```python
from build123d import *

# Parameters (mm, degrees)
RESSALTO_EXTRUS_O1_DEPTH = 12.5


with BuildPart() as part:
    # Esboço1 → Ressalto-extrusão1 (new body)
    with BuildSketch(Plane.XY):
        with BuildLine():
            Line((10, -22.912878475), (10, -17.320508076))
            ThreePointArc((10, -17.320508076), (-19.318516526, -5.176380902), (0, 20))
            Line((0, 20), (0, 40))
            ThreePointArc((0, 40), (-2.5, 42.5), (-5, 40))
            Line((-5, 40), (-4.923076923, 39.384615385))
            Line((-4.923076923, 39.384615385), (-2.728764161, 21.830113288))
            ThreePointArc((-2.728764161, 21.830113288), (-21.36959311, 5.228813472), (-12.5, -18.10386699))
            Line((-12.5, -18.10386699), (-12.5, -21.650635095))
            ThreePointArc((-12.5, -21.650635095), (-1.400290894, -24.960752902), (10, -22.912878475))
        make_face()
    extrude(amount=RESSALTO_EXTRUS_O1_DEPTH)


solid = part.part
```
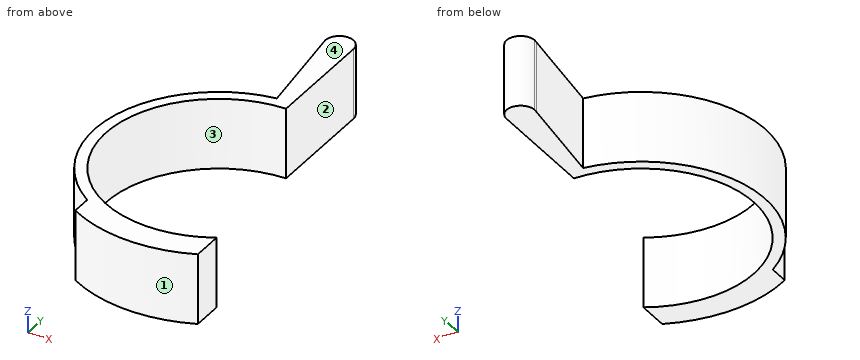
Read the model definition and answer for the solid it produces. Units are mm, in the model's axes. Face numbers are marked on the shaded views. Give positions to 0.01 mm unless a question says otherwise; leave off trailing zeros. Loops run counter-clockwise (first coordinate to the right, second up) from the corner with the lowest first, then second, coordinate; pieces in that order, holes last.
Item 1: The part is cut by section B-B (z = 4). Write down the section's boundary in (x, y), and give its area (3 significant figures).
Item 2: The part is cut by section C-C (y = 0). Write down the section's boundary in (x, z), and give its area (3 significant figures).
Item 3: The part is cut by section A-A (x = -6). Write down the section's boundary in (y, z), and give its area (3 significant figures).
Item 4: The part is cut by section D-D (x = -1). Write down the section's boundary in (y, z).
Item 5: The mould has two halves that part along X. Classify the marked faces 1, 2, 3 and 4: released by +X, released by -X, zero draft, split by the parting line, or undercut.
Item 6: Find the intervals of material crossed by line 1 along X through (y, z) = (0, 3.75); line 2 along Y through (x, z) = (-18, 7); line 3 along X through (y, z) = (38, 2.75), in increasing order.
Item 7: Each of these flat-tipped pins is pushed along its axis until it touches: pin 1 Ø4 at (y, z) = (-18, 10) entering from -X; pin 2 Ø1.1 at (y, z) = (-20.5, 4) entering from -X; pin 3 Ø4 at (x, z) = (-18, 8.5) entering from -Y. Where does it stop, or does it pass through?
Taken from the geometry:
1. outline: (-12.5, -21.65) arc R25 ccw to (10, -22.91) - (10, -17.32) arc R20 cw (long way) to (0, 20) - (0, 40) arc R2.5 ccw to (-5, 40) - (-2.73, 21.83) arc R22 ccw to (-12.5, -18.1) - close
1. area: 303 mm2
2. outline: (-22, 0) - (-20, 0) - (-20, 12.5) - (-22, 12.5) - close
2. area: 25.0 mm2
3. outline: (-24.27, 0) - (-19.08, 0) - (-19.08, 12.5) - (-24.27, 12.5) - close; (19.08, 0) - (21.17, 0) - (21.17, 12.5) - (19.08, 12.5) - close
3. area: 91.0 mm2
4. outline: (-24.98, 0) - (-19.97, 0) - (-19.97, 12.5) - (-24.98, 12.5) - close; (19.97, 0) - (42, 0) - (42, 12.5) - (19.97, 12.5) - close
5. face 1: split by the parting line
5. face 2: released by +X
5. face 3: undercut
5. face 4: zero draft
6. line 1: x = -22 to -20
6. line 2: y = -12.65 to -8.72, 8.72 to 12.65
6. line 3: x = -4.75 to 0
7. pin 1: stops at x = -15.1
7. pin 2: stops at x = -12.5
7. pin 3: stops at y = -15.1
